```python
from build123d import *

# Parameters (mm, degrees)
SKETCH_W        = 90
SKETCH_H        = 105
PAD_DEPTH       = 50
POCKET_DEPTH    = 48.4
PAD001_DEPTH    = 105
PAD002_DEPTH    = 90
PAD003_DEPTH    = 6.6
SKETCH008_R     = 1
POCKET004_DEPTH = 5
POCKET001_DEPTH = 105.001
POCKET002_DEPTH = 90.001
POCKET003_DEPTH = 50.001


with BuildPart() as part:
    # Sketch → Pad (new body)
    with BuildSketch(Plane.XY):
        Rectangle(SKETCH_W, SKETCH_H)
    extrude(amount=PAD_DEPTH)

    # Sketch001 (on DatumPlane) → Pocket (cut)
    with BuildSketch(Plane.XY.offset(50)):
        with BuildLine():
            Line((-43, 50.9), (43, 50.9))
            ThreePointArc((43.4, 50.5), (43.282843, 50.782843), (43, 50.9))
            Line((43.4, 50.5), (43.4, -50.5))
            ThreePointArc((43, -50.9), (43.282843, -50.782843), (43.4, -50.5))
            Line((43, -50.9), (-43, -50.9))
            ThreePointArc((-43.4, -50.5), (-43.282843, -50.782843), (-43, -50.9))
            Line((-43.4, -50.5), (-43.4, 50.5))
            ThreePointArc((-43, 50.9), (-43.282843, 50.782843), (-43.4, 50.5))
        make_face()
    extrude(amount=-POCKET_DEPTH, mode=Mode.SUBTRACT)

    # Sketch002 (on DatumPlane) → Pad001 (join)
    with BuildSketch(Plane.XZ.offset(52.5)):
        Polygon((-45, 4.666905), (-40.333095, 0), (-45, 0), align=None)
        Polygon((40.333095, 0), (45, 0), (45, 4.666905), align=None)
    extrude(amount=-PAD001_DEPTH)

    # Sketch003 (on DatumPlane) → Pad002 (join)
    with BuildSketch(Plane.YZ.offset(45)):
        Polygon((-52.5, 4.666905), (-52.5, 0), (-47.833095, 0), align=None)
        Polygon((47.833095, 0), (52.5, 0), (52.5, 4.666905), align=None)
    extrude(amount=-PAD002_DEPTH)

    # Sketch007 → Pad003 (join)
    with BuildSketch(Plane.XY):
        with BuildLine():
            ThreePointArc((-40, 42.5), (-36.464466, 43.964466), (-35, 47.5))
            Line((-35, 52.5), (-35, 47.5))
            Line((-35, 52.5), (-45, 52.5))
            Line((-45, 52.5), (-45, 42.5))
            Line((-40, 42.5), (-45, 42.5))
        make_face()
        with BuildLine():
            ThreePointArc((35, 47.5), (36.464466, 43.964466), (40, 42.5))
            Line((45, 42.5), (40, 42.5))
            Line((45, 52.5), (45, 42.5))
            Line((45, 52.5), (35, 52.5))
            Line((35, 52.5), (35, 47.5))
        make_face()
        with BuildLine():
            ThreePointArc((40, -42.5), (36.464466, -43.964466), (35, -47.5))
            Line((35, -47.5), (35, -52.5))
            Line((45, -52.5), (35, -52.5))
            Line((45, -42.5), (45, -52.5))
            Line((45, -42.5), (40, -42.5))
        make_face()
        with BuildLine():
            ThreePointArc((-35, -47.5), (-36.464466, -43.964466), (-40, -42.5))
            Line((-40, -42.5), (-45, -42.5))
            Line((-45, -42.5), (-45, -52.5))
            Line((-45, -52.5), (-35, -52.5))
            Line((-35, -47.5), (-35, -52.5))
        make_face()
    extrude(amount=PAD003_DEPTH)

    # Sketch008 → Pocket004 (cut)
    with BuildSketch(Plane.XY):
        with Locations((-40, 47.5)):
            Circle(SKETCH008_R)
        with Locations((40, 47.5)):
            Circle(SKETCH008_R)
        with Locations((40, -47.5)):
            Circle(SKETCH008_R)
        with Locations((-40, -47.5)):
            Circle(SKETCH008_R)
    extrude(amount=POCKET004_DEPTH, mode=Mode.SUBTRACT)

    # Sketch004 (on DatumPlane) → Pocket001 (cut, through all)
    with BuildSketch(Plane.XZ.offset(52.5)):
        Polygon((-45, 0), (-45, 3.535534), (-41.464466, 0), align=None)
        Polygon((41.464466, 0), (45, 0), (45, 3.535534), align=None)
    extrude(amount=-POCKET001_DEPTH, mode=Mode.SUBTRACT)

    # Sketch005 (on DatumPlane) → Pocket002 (cut, through all)
    with BuildSketch(Plane.YZ.offset(45)):
        Polygon((-52.5, 0), (-52.5, 3.535534), (-48.964466, 0), align=None)
        Polygon((48.964466, 0), (52.5, 0), (52.5, 3.535534), align=None)
    extrude(amount=-POCKET002_DEPTH, mode=Mode.SUBTRACT)

    # Sketch006 (on DatumPlane) → Pocket003 (cut, through all)
    with BuildSketch(Plane.XY.offset(50)):
        with BuildLine():
            ThreePointArc((-43, 52.5), (-44.414214, 51.914214), (-45, 50.5))
            Line((-45, 52.5), (-45, 50.5))
            Line((-43, 52.5), (-45, 52.5))
        make_face()
        with BuildLine():
            ThreePointArc((45, 50.5), (44.414214, 51.914214), (43, 52.5))
            Line((43, 52.5), (45, 52.5))
            Line((45, 50.5), (45, 52.5))
        make_face()
        with BuildLine():
            ThreePointArc((43, -52.5), (44.414214, -51.914214), (45, -50.5))
            Line((45, -52.5), (45, -50.5))
            Line((43, -52.5), (45, -52.5))
        make_face()
        with BuildLine():
            ThreePointArc((-45, -50.5), (-44.414214, -51.914214), (-43, -52.5))
            Line((-45, -52.5), (-43, -52.5))
            Line((-45, -50.5), (-45, -52.5))
        make_face()
    extrude(amount=-POCKET003_DEPTH, mode=Mode.SUBTRACT)


solid = part.part
```
Model file for the job. Use its own axes, mm. A direction names the side the tool comes from. Coordinates: 2 decimals unless noted, no trailing zeros. Loops run counter-clockwise (first coordinate to the right, second up) from the corner with the lowest first, then second, coordinate; pieces in that order, holes last. Notation, with made-up numbers: (71.5, 3) - (119.5, 3) arc R16 ccw to (119.5, 31) - close; hole circle Ø7 at (14.25, 5). An arc over 180 degrees is marked (long way). Answer as a JSON object with one key per item and string values. Group by question number.
(1) Flat gauge pins, fed straight in: pin 1 (5 mm diameter, centred on x = 7, y = -24.5, fed in from +Z); pin 2 (1.6 mm diameter, centred on x = 40.5, y = 47.5, fed in from -Z); pin 3 (1 mm diameter, centred on y = -50, z = 3, fed in from +X); pin 4 (0.6 mm diameter, centred on x = -40, y = -47.5, fed in from -Z). Where does each tip first touch, or does it go through?
(2) Cut at A-A (y = -25.5). Give the cut face in (x, z).
(3) Cut at B-B (z = 9). Give the cut face in (x, y).
(4) Probe line 1 along Y through (x, z) = (-40, 4); line 2 along X through (y, z) = (-25.5, 11); line 3 along X through (y, z) = (-47, 1). List the from-to ranges inside material, lowest first.
(5) Two-plate mould, pull along Y, no slides. Class faces 3 (the face through (43.4, 1, 27)), 4 (the face through (-36.43, -44, 4.07)), 5 (the face through (43.257, -0.727, 1.793)), 6 (the face through (-1, -52.5, 26)): released by +Y, released by -Y, zero draft, split by the parting line, or undercut.
(6) Tool access for faces 1 (the face through (-39, -47, 6.6)), 2 (the face through (-43.257, -0.727, 1.793)): list every direction of +Z, -Z, +X, -X, +Y, -Y with a clear straight run to the whole face (end or side of a thin tool).
(7) Cut at C-C (x = -18.5). Give the cut face in (y, z), then the cut area to 3 significant figures.
Geometry says:
{
 "1": {"pin 1": "stops at z = 1.6", "pin 2": "stops at z = 0", "pin 3": "stops at x = 44.96", "pin 4": "stops at z = 5"},
 "2": {"outline": "(-45, 3.54) - (-41.46, 0) - (41.46, 0) - (45, 3.54) - (45, 50) - (43.4, 50) - (43.4, 3.07) - (41.93, 1.6) - (-41.93, 1.6) - (-43.4, 3.07) - (-43.4, 50) - (-45, 50) - close"},
 "3": {"outline": "(-45, -50.5) arc R2 ccw to (-43, -52.5) - (43, -52.5) arc R2 ccw to (45, -50.5) - (45, 50.5) arc R2 ccw to (43, 52.5) - (-43, 52.5) arc R2 ccw to (-45, 50.5) - close; hole (-43.4, -50.5) arc R0.4 ccw to (-43, -50.9) - (43, -50.9) arc R0.4 ccw to (43.4, -50.5) - (43.4, 50.5) arc R0.4 ccw to (43, 50.9) - (-43, 50.9) arc R0.4 ccw to (-43.4, 50.5) - close"},
 "4": {"line 1": "y = -52.5 to -48.5, -46.5 to -42.5, 42.5 to 46.5, 48.5 to 52.5", "line 2": "x = -45 to -43.4, 43.4 to 45", "line 3": "x = -42.46 to -40.87, -39.13 to 39.13, 40.87 to 42.46"},
 "5": {"face 3": "undercut", "face 4": "undercut", "face 5": "zero draft", "face 6": "released by -Y"},
 "6": {"face 1": "+Z", "face 2": "-Z, -X, +Y, -Y"},
 "7": {"outline": "(-52.5, 3.54) - (-48.96, 0) - (48.96, 0) - (52.5, 3.54) - (52.5, 50) - (50.9, 50) - (50.9, 3.07) - (49.43, 1.6) - (-49.43, 1.6) - (-50.9, 3.07) - (-50.9, 50) - (-52.5, 50) - close", "area": "313 mm^2"}
}
